from build123d import *

# Parameters (mm, degrees)
SKETCH1_W           = 150
SKETCH1_H           = 5
BOSS_EXTRUDE1_DEPTH = 50
SKETCH2_W           = 15
SKETCH2_H           = 10
BOSS_EXTRUDE2_DEPTH = 50
SKETCH3_W           = 95
SKETCH3_H           = 5
BOSS_EXTRUDE3_DEPTH = 60
SKETCH4_W           = 50
SKETCH4_H           = 30
BOSS_EXTRUDE4_DEPTH = 17
BOSS_EXTRUDE5_DEPTH = 95
FILLET1_R           = 7.5
SKETCH6_R           = 3.5
CUT_EXTRUDE1_DEPTH  = 30
CUT_EXTRUDE2_DEPTH  = 10
CUT_EXTRUDE3_DEPTH  = 10
SCALE1_SCALE        = 2
SCALE4_SCALE        = 0.5


with BuildPart() as part:
    # Sketch1 → Boss-Extrude1 (new body)
    with BuildSketch(Plane.XY):
        with Locations((75, 2.5)):
            Rectangle(SKETCH1_W, SKETCH1_H)
    extrude(amount=-BOSS_EXTRUDE1_DEPTH)

    # Sketch2 → Boss-Extrude2 (add)
    with BuildSketch(Plane(origin=(0, 5, 0), x_dir=(1, 0, 0), z_dir=(0, 1, 0))):
        with Locations((7.5, 25)):
            Rectangle(SKETCH2_W, SKETCH2_H)
    extrude(amount=BOSS_EXTRUDE2_DEPTH)

    # Sketch3 → Boss-Extrude3 (add)
    with BuildSketch(Plane(origin=(0, 5, 0), x_dir=(1, 0, 0), z_dir=(0, 1, 0))):
        with Locations((102.5, 47.5)):
            Rectangle(SKETCH3_W, SKETCH3_H)
    extrude(amount=BOSS_EXTRUDE3_DEPTH)

    # Sketch4 → Boss-Extrude4 (add)
    with BuildSketch(Plane(origin=(0, 5, 0), x_dir=(1, 0, 0), z_dir=(0, 1, 0))):
        with Locations((125, 15)):
            Rectangle(SKETCH4_W, SKETCH4_H)
    extrude(amount=BOSS_EXTRUDE4_DEPTH)

    # Sketch5 → Boss-Extrude5 (add)
    with BuildSketch(Plane(origin=(150, 0, 0), x_dir=(0, 0, -1), z_dir=(1, 0, 0))):
        Polygon((45, 65), (40, 65), (40, 59), (45, 61), align=None)
        Polygon((45, 19), (40, 19), (40, 25), (45, 23), align=None)
    extrude(amount=-BOSS_EXTRUDE5_DEPTH)

    # Fillet1
    fillet1_edges = [part.edges().sort_by_distance(p)[0] for p in [
        (15, 55, -25),
        (0, 55, -25),
    ]]
    fillet(fillet1_edges, radius=FILLET1_R - 0.0001)  # a hair under: the kernel refuses the full size

    # Sketch6 → Cut-Extrude1 (cut)
    with BuildSketch(Plane.XY.offset(-20)):
        with Locations((7.5, 47.5)):
            Circle(SKETCH6_R)
    extrude(amount=-CUT_EXTRUDE1_DEPTH, mode=Mode.SUBTRACT)

    # Sketch7 → Cut-Extrude2 (cut)
    with BuildSketch(Plane.XY.offset(-45)):
        with BuildLine():
            Line((75, 55), (123, 55))
            ThreePointArc((123, 55), (125, 53), (123, 51))
            Line((123, 51), (75, 51))
            ThreePointArc((75, 51), (73, 53), (75, 55))
        make_face()
    extrude(amount=-CUT_EXTRUDE2_DEPTH, mode=Mode.SUBTRACT)

    # Sketch8 → Cut-Extrude3 (cut)
    with BuildSketch(Plane.XY.offset(-45)):
        with BuildLine():
            Line((77, 53), (77, 31))
            ThreePointArc((77, 31), (75, 29), (73, 31))
            Line((73, 31), (73, 53))
            ThreePointArc((73, 53), (75, 55), (77, 53))
        make_face()
    extrude(amount=-CUT_EXTRUDE3_DEPTH, mode=Mode.SUBTRACT)


with BuildPart() as part_1:
    # Scale1: scaled about (91.729979694, 17.282886664, -29.286286863)
    add(part.part.scale(SCALE1_SCALE).moved(Location((-91.729979694, -17.282886664, 29.286286863))))


with BuildPart() as part_2:
    # Scale4: scaled about (91.729979694, 17.282886664, -29.286286864)
    add(part_1.part.scale(SCALE4_SCALE).moved(Location((45.864989847, 8.641443332, -14.643143432))))


solid = part_2.part
Build history of the part. All positions in model axes, mm. A direction names the side the tool comes from. Round coordinates to 2 decimals unless told otherwise and drop trailing zeros. Loops run counter-clockwise (first coordinate to the right, second up) from the corner with the lowest first, then second, coordinate; pieces in that order, holes last. Notation, with made-up numbers: (54, 45) -> (90, 45) arc R27 ccw to (90, 83) -> close; hole circle Ø1 at (-39.5, 40.5). An arc over 180 degrees is marked (long way). Use CSV: the item, a comma, the result in double quotes. Start each with the question number.
Q1. Saw through at B-B on x = 117.5. Give the cut face in (y, z).
Q2. Drill centre lines: L1, parallel to X at y = 13, z = -23; L2, parallel to Y at x = 122.5, z = -43; L3, parallel to Y at x = 7.5, z = -24.75. Where is each one in solid material? Low to high.
Q3. Mould opens along Z. For faces 1 (the face through (125, 53, -47)), 2 (the face through (7, 30, -20)), 3 (the face through (103.2, 24, -42.5)), 4 (the face through (91, 25, -50)) say: +Z half, -Z half, draft (parallel to the pull), parting line (faces both ways), or undercut.
Q4. Flat gauge pins, fed straight in: pin 1 Ø3 at (x, y) = (69.5, 14.5) entering from +Z; pin 2 Ø4 at (y, z) = (40, -48.5) entering from -X; pin 3 Ø11 at (y, z) = (34.5, -26) entering from +X; pin 4 Ø5 at (y, z) = (28, -15.5) entering from +X. Where does each tip first touch, or does it go through?
Q5. Saw through at C-C on y = 27.5. Give the cut face in (x, z), and give its area (3 significant figures).
Q6. Which spindle directions (+Z, -Z, +X, -X, +Y, -Y) get a long thin tool onto all of the face, cutting with end or side? Do faces 5 (the face through (15, 26, -25)), 6 (the face through (103.2, 60, -42.5)), 7 (the face through (73, 42, -47)). Say none if no direction does.
Q7. Saw through at D-D on z = -14. Give the cut face in (x, y).
Q8. Saw through at A-A on y = 35. Give the cut face in (x, z), and give its area (3 significant figures).
Solutions:
1,outline,"(0, -50) -> (51, -50) -> (51, -45) -> (23, -45) -> (25, -40) -> (19, -40) -> (19, -45) -> (5, -45) -> (5, -30) -> (22, -30) -> (22, 0) -> (0, 0) -> close; (55, -50) -> (65, -50) -> (65, -40) -> (59, -40) -> (61, -45) -> (55, -45) -> close"
2,L1,"x = 0 to 15, 100 to 150"
2,L2,"y = 0 to 5, 19 to 23.8, 60.2 to 65"
2,L3,"y = 0 to 44, 51 to 55"
3,face 1,"draft"
3,face 2,"+Z half"
3,face 3,"undercut"
3,face 4,"-Z half"
4,pin 1,"stops at z = -45"
4,pin 2,"stops at x = 55"
4,pin 3,"stops at x = 15"
4,pin 4,"passes through"
5,outline,"(0, -30) -> (15, -30) -> (15, -20) -> (0, -20) -> close; (55, -50) -> (150, -50) -> (150, -45) -> (55, -45) -> close"
5,area,"625 mm^2"
6,face 5,"+Z, -Z, +Y"
6,face 6,"+X, -X"
6,face 7,"+Z, -Z"
7,outline,"(0, 0) -> (150, 0) -> (150, 22) -> (100, 22) -> (100, 5) -> (0, 5) -> close"
8,outline,"(0, -30) -> (15, -30) -> (15, -20) -> (0, -20) -> close; (55, -50) -> (73, -50) -> (73, -45) -> (55, -45) -> close; (77, -50) -> (150, -50) -> (150, -45) -> (77, -45) -> close"
8,area,"605 mm^2"
